from build123d import *

# Parameters (mm, degrees)
SKETCH1_R           = 9
BOSS_EXTRUDE1_DEPTH = 10
BOSS_EXTRUDE1_TAPER = 35
SKETCH2_R           = 9
BOSS_EXTRUDE2_DEPTH = 10
BOSS_EXTRUDE2_DRAFT = 45
SKETCH3_R           = 4
CUT_EXTRUDE1_DEPTH  = 20


with BuildPart() as part:
    # Sketch1 → Boss-Extrude1 (new body)
    with BuildSketch(Plane.XY):
        Circle(SKETCH1_R)
    extrude(amount=BOSS_EXTRUDE1_DEPTH, taper=BOSS_EXTRUDE1_TAPER)


with BuildPart() as boss_extrude2_tool:
    # Sketch2 → Boss-Extrude2 (with draft: the straight prism first)
    with BuildSketch(Plane(origin=(0, 0, 10), x_dir=(-1, 0, 0), z_dir=(0, 0, -1))):
        Circle(SKETCH2_R)
    extrude(amount=BOSS_EXTRUDE2_DEPTH)
    # Boss-Extrude2: the draft: its side faces are tilted about the plane it starts from
    boss_extrude2_sides = [boss_extrude2_tool.faces().sort_by_distance(p)[0] for p in [
        (9, 0, 5),
    ]]
    draft(boss_extrude2_sides, Plane(origin=(0, 0, 10), x_dir=(-1, 0, 0), z_dir=(0, 0, -1)), BOSS_EXTRUDE2_DRAFT)


with BuildPart() as part_1:
    add(part.part)

    # Boss-Extrude2: add boss_extrude2_tool
    add(boss_extrude2_tool.part)

    # Sketch3 → Cut-Extrude1 (cut)
    with BuildSketch(Plane(origin=(0, 0, 10), x_dir=(-1, 0, 0), z_dir=(0, 0, -1))):
        Circle(SKETCH3_R)
    extrude(amount=CUT_EXTRUDE1_DEPTH, mode=Mode.SUBTRACT)


solid = part_1.part
The model under review builds one solid part; all positions refer to its coordinate system, in mm. Give positions to 0.01 mm unless a question says otherwise; leave off trailing zeros. Order: outer loops, then holes, each group sorted by start corner. A loop starts at its lowest first (then second) coordinate and runs counter-clockwise, first axis right, second up. Notation, with made-up numbers: M -27,78.25 L 10,78.25 A27 cw 10,113.25 Z; hole C 19,-6 d2. An arc over 180 degrees is marked long. Answer in a Markdown table with one row per item. Add a question column.
1. For pin 1 Ø3 at (x, z) = (-3, 2.5) entering from -Y; pin 2 Ø5 at (y, z) = (-1, 3) entering from +X; pin 3 Ø5 at (y, z) = (6.5, 3) entering from -X; pin 4 Ø6 at (x, y) = (5, -2) entering from -Z, all flat-tipped, find the tip position at first contact; note any pin that passes through.
2. To check wall thickness, follow line 1 along Y through (x, z) = (0, 3.5); line 2 along Z through (x, y) = (7, -4); line 3 along Y through (x, z) = (-1, 7.25). State the ranges of each line that lie inside material, in increasing order.
3. Mouldability with a two-part tool opening along Z and no side actions: class faces 1 (the conical face through (1.11, -5.02, 6.14)), 2 (the conical face through (4.69, -1.95, 5.6)), 3 (the flat face through (-4, -2, 10)), 4 (the cylindrical face through (0.867, -3.905, 5.07)) as released by +Z, released by -Z, zero draft, split by the parting line, or undercut.
4. Add section B-B on z = 8. State the section outline as (x, y) points.
5. Add section A-A on x = 0. State the section outline as (y, z) points, plus the area to 3 significant figures.
6. Add section D-D on z = 3. State the section outline as (x, y) points, plus the area to 3 significant figures.
The answers:
| question | item | result |
|---|---|---|
| 1 | pin 1 | y = -7.85 |
| 1 | pin 2 | x = 8.61 |
| 1 | pin 3 | x = -6.63 |
| 1 | pin 4 | z = 0 |
| 2 | line 1 | -6.55 to -4, 4 to 6.55 |
| 2 | line 2 | 0 to 1.34, 9.06 to 10 |
| 2 | line 3 | -6.17 to -3.87, 3.87 to 6.17 |
| 3 | face 1 | undercut |
| 3 | face 2 | undercut |
| 3 | face 3 | released by +Z |
| 3 | face 4 | zero draft |
| 4 | outline | C 0,0 d14; hole C 0,0 d8 |
| 5 | outline | M -9,0 L -4,0 L -4,10 L -9,10 L -4.88,5.88 Z; M 4,0 L 9,0 L 4.88,5.88 L 9,10 L 4,10 Z |
| 5 | area | 58.8 mm2 |
| 6 | outline | C 0,0 d13.8; hole C 0,0 d8 |
| 6 | area | 99.3 mm2 |
